Could you check a few things on this model? Use its own coordinates, in mm. A direction names the side the tool comes from. Coordinates: 2 decimals unless noted, no trailing zeros. Loops run counter-clockwise (first coordinate to the right, second up) from the corner with the lowest first, then second, coordinate; pieces in that order, holes last. Notation, with made-up numbers: M -24,89 L 28,89 A30 cw 28,120 Z; hole C 47,-19 d10. An arc over 180 degrees is marked long. Write each question's results on one line, items separated by ' | '.
Autodesk Inventor part; units mm, degrees
ref_plane "YZ Plane" through (0, 0, 0) normal (1, 0, 0) x (0, 1, 0)
ref_plane "XZ Plane" through (0, 0, 0) normal (0, 1, 0) x (-1, 0, 0)
ref_plane "XY Plane" through (0, 0, 0) normal (0, 0, 1) x (1, 0, 0)
sketch "スケッチ1" plane through (0, 0, 0) normal (0, 0, 1) x (1, 0, 0)
  circle A0 centre (0, 0) radius 5
  circle A1 centre (0, 35) radius 5
  line L0 (0, 35) -> (0, 0)
  arc A2 (0.9687, -4.9053) -> (0.9687, 39.9053) centre (-3.456, 17.5) ccw
  arc A3 (-0.9687, 4.9053) -> (-0.9687, 30.0947) centre (-3.456, 17.5) ccw
  point P0 (0, 30)
  point P1 (0, 29.8641)
  point P2 (0, 5.1359)
  point P3 (0, 5)
  dimension "d0" = 10
  dimension "d1" = 10
  dimension "d2" = 35
  dimension "d3" = 22.838
  dimension "d4" = 12.838
extrude "押し出し1" add sketch "スケッチ1" along normal blind 5 contours A0 | A3 L0 A0 | A0 L0 A3 A1 A2 | A1 | A3 A1 L0
sketch "スケッチ2" plane through (0, 0, 0) normal (0, 0, -1) x (-1, 0, 0)
  circle A0 centre (0, 0) radius 5
extrude "押し出し2" add sketch "スケッチ2" along normal blind 5.6
sketch "スケッチ3" plane through (0, 0, -5.6) normal (0, 0, -1) x (-1, 0, 0)
  circle A0 centre (0, 0) radius 3.1
  dimension "d9" = 6.2
extrude "押し出し3" cut sketch "スケッチ3" against normal blind 2.5
sketch "スケッチ4" plane through (0, 0, 5) normal (0, 0, 1) x (1, 0, 0)
  circle A0 centre (0, 0) radius 3.1
  arc A1 (0.9687, 39.9053) -> (-0.9687, 30.0947) centre (0, 35) ccw
  point P0 (0, 30)
hole "穴1" at (0, 0, 5) at (0, 35, 5) direction (0, 0, -1) diameter 3.6 end through all
sketch "スケッチ5" plane through (0, 0, 0) normal (0, 0, -1) x (-1, 0, 0)
  circle A0 centre (0, 35) radius 1.8
  circle A1 centre (0, 35) radius 3.7
  point P0 (0, 0)
  dimension "d19" = 7.4
extrude "押し出し4" cut sketch "スケッチ5" against normal blind 0.6
sketch "スケッチ7" plane through (0, 0, 5) normal (0, 0, 1) x (1, 0, 0)
  circle A0 centre (0, 35) radius 1.8
  point P0 (0, 0)
hole "穴3" at (0, 35, 5) direction (0, 0, -1) diameter 6.2 end through all
fillet "フィレット2" radius 0.5 1 edges at (3.7, 35, 0)
fillet "フィレット3" radius 0.1 1 edges at (0, 38.1, 0.6)
sketch "スケッチ8" plane through (0, 0, 5) normal (0, 0, 1) x (1, 0, 0)
  circle A0 centre (0, 0) radius 1.8
  circle A1 centre (0, 0) radius 3.1
  dimension "d39" = 6.2
extrude "押し出し5" cut sketch "スケッチ8" against normal blind 2.5
sketch "スケッチ10" plane through (0, 0, 5) normal (0, 0, 1) x (1, 0, 0)
  circle A0 centre (0, 35) radius 3.1
  circle A1 centre (0, 35) radius 3.7
  point P0 (0, 0)
  dimension "d45" = 7.4
extrude "押し出し7" cut sketch "スケッチ10" against normal blind 0.6 contours A0 | A1
fillet "フィレット4" radius 0.2 2 edges at (0, 38.1, 4.4) (-3.7, 35, 5)
properties part number "rotor_arm_ver2" material "アルミニウム 6061"
(1) Which directions (+Z, -Z, +X, -X, +Y, -Y) give clear straight access to the entire face, cutting with the end or side of a thin tool? Please do faces 5 (the flat face through (-2, 0, -3.1)), 6 (the cylindrical face through (-0.541, -1.717, -0.339)), 7 (the cylindrical face through (1.43, -2.75, 3.77)).
Reported:
face 5: -Z | face 6: +Z, -Z | face 7: +Z
(2) Imagine slicing it at A-A, the plane y = 35. List the corners of the cut face in (x, z) for me, and give its area (3 significant figures).
Reported:
outline: M -5,0 L -4.2,0 A0.5 ccw -3.7,0.5 L -3.7,0.6 L -3.2,0.6 A0.1 ccw -3.1,0.7 L -3.1,4.2 A0.2 ccw -3.3,4.4 L -3.7,4.4 L -3.7,4.8 A0.2 ccw -3.9,5 L -5,5 Z; M 3.1,0.7 A0.1 ccw 3.2,0.6 L 3.7,0.6 L 3.7,0.5 A0.5 ccw 4.2,0 L 11.22,0 L 11.22,5 L 3.9,5 A0.2 ccw 3.7,4.8 L 3.7,4.4 L 3.3,4.4 A0.2 ccw 3.1,4.2 Z | area: 48.5 mm2
(3) Imagine slicing it at B-B, the plane z = -1.75. List the corners of the cut face in (x, y) for me.
Reported:
outline: C 0,0 d10; hole C 0,0 d3.6
(4) Will these pins go through, and if not, where does the flat tip stop? P1, Ø8, axis at x = -0.5, y = 35.5, coming from the +Z side; P2, Ø12, axis at x = 7, y = 11, coming from the -Z side; P3, Ø4, axis at x = 0, y = 0, coming from the +Z side; P4, Ø5, axis at y = 20.5, z = 1, coming from the -X side.
Reported:
P1: stops at z = 5 | P2: stops at z = 0 | P3: stops at z = 2.5 | P4: stops at x = 8.14
(5) If we mould it in two halves opening along X, with no side actions, what happens to faces 1 (the flat face through (2, 0, 2.5)), 2 (the cylindrical face through (-4.44, 2.3, 0.95)), 3 (the cylindrical face through (9.38, 17.75, 2.46)), 4 (the flat face through (10, 18, 0))? For each: released by +X, released by -X, zero draft, split by the parting line, or undercut.
Reported:
face 1: undercut | face 2: split by the parting line | face 3: released by -X | face 4: zero draft
(6) Please list where these lines run through material, in increasing order: probe 1 along Y at (x, z) = (0, 4.75); probe 2 along Y at (x, z) = (0, -1.85); probe 3 along Y at (x, z) = (-2.5, 2.75). Write a range as from..to.
Reported:
probe 1: y = -5..-3.1, 3.1..5.14, 29.86..31.3, 38.7..40 | probe 2: y = -5..-1.8, 1.8..5 | probe 3: y = -4.33..-1.83, 1.83..4.33, 30.67..33.17, 36.83..39.33
(7) Imagine slicing it at D-D, the plane x = 0. State how many separate pieces and enclosed holes the cut face has, and give its area (3 significant figures).
Reported:
separate pieces: 4 | enclosed holes: 0 | area: 73.6 mm2
